from build123d import *

# Parameters (mm, degrees)
SKETCH1_W           = 33
SKETCH1_H           = 28
BOSS_EXTRUDE1_DEPTH = 46
CUT_EXTRUDE1_DEPTH  = 59.318093247
CUT_EXTRUDE2_START  = -3
CUT_EXTRUDE2_DEPTH  = 27
FILLET2_R           = 12.5
FILLET3_R           = 16.5
FILLET4_R           = 6
SKETCH5_W           = 13
SKETCH5_H           = 23
CUT_EXTRUDE3_DEPTH  = 9
SKETCH6_R           = 6.5
CUT_EXTRUDE4_DEPTH  = 56.592265809
SKETCH7_R           = 1
CUT_EXTRUDE6_DEPTH  = 8
SKETCH8_R           = 1.3
SKETCH8_R_2         = 2.5
CUT_EXTRUDE7_DEPTH  = 2.5


with BuildPart() as part:
    # Sketch1 → Boss-Extrude1 (new body)
    with BuildSketch(Plane.XY):
        Rectangle(SKETCH1_W, SKETCH1_H)
    extrude(amount=BOSS_EXTRUDE1_DEPTH)

    # Sketch2 → Cut-Extrude1 (cut, through all)
    with BuildSketch(Plane(origin=(16.5, 0, 0), x_dir=(0, 0, -1), z_dir=(1, 0, 0))):
        with BuildLine():
            Line((-46, 2), (-46, -14))
            Line((-46, -14), (-5, -14))
            add(Edge.make_bspline(
                [(-5, -14), (-24.903930892, -4.26145895), (-46, 2)],
                knots=[0, 0, 0, 1, 1, 1], degree=2))
        make_face()
    extrude(amount=-CUT_EXTRUDE1_DEPTH, mode=Mode.SUBTRACT)

    # Sketch4 → Cut-Extrude2 (cut)
    with BuildSketch(Plane(origin=(16.5, 0, 0), x_dir=(0, 0, -1), z_dir=(1, 0, 0)).offset(CUT_EXTRUDE2_START)):
        with BuildLine():
            Line((-5, -14), (-2.5, -14))
            Line((-2.5, -14), (-2.5, 3.5))
            Line((-2.5, 3.5), (-40.5, 3.5))
            Line((-40.5, 3.5), (-40.5, 0.301980422))
            add(Edge.make_bspline(
                [(-5, -14), (-22.299705813, -5.535647097), (-40.5, 0.301980422)],
                knots=[0, 0, 0, 1, 1, 1], degree=2))
        make_face()
    extrude(amount=-CUT_EXTRUDE2_DEPTH, mode=Mode.SUBTRACT)

    # Fillet2
    fillet2_edges = [part.edges().sort_by_distance(p)[0] for p in [
        (-13.5, 1.900990211, 40.5),
        (13.5, 1.900990211, 40.5),
    ]]
    fillet(fillet2_edges, radius=FILLET2_R)

    # Fillet3
    fillet3_edges = [part.edges().sort_by_distance(p)[0] for p in [
        (-16.5, 8, 46),
        (16.5, 8, 46),
    ]]
    fillet(fillet3_edges, radius=FILLET3_R - 0.0001)  # a hair under: the kernel refuses the full size

    # Fillet4
    fillet4_edges = [part.edges().sort_by_distance(p)[0] for p in [
        (-16.5, -14, 2.5),
        (16.5, -14, 2.5),
    ]]
    fillet(fillet4_edges, radius=FILLET4_R)

    # Sketch5 → Cut-Extrude3 (cut)
    with BuildSketch(Plane.XZ.offset(-3.5)):
        with Locations((0, 20.5)):
            Rectangle(SKETCH5_W, SKETCH5_H)
    extrude(amount=-CUT_EXTRUDE3_DEPTH, mode=Mode.SUBTRACT)

    # Sketch6 → Cut-Extrude4 (cut, through all)
    with BuildSketch(Plane.XZ.offset(-12.5)):
        with Locations(Location((0, 25.5, 0), (0, 0, 270))):
            Circle(SKETCH6_R)
    extrude(amount=-CUT_EXTRUDE4_DEPTH, mode=Mode.SUBTRACT)

    # Sketch7 → Cut-Extrude6 (cut)
    with BuildSketch(Plane.XZ.offset(-3.5)):
        with Locations(Location((0, 34.052667497, 0), (0, 0, 270))):
            Circle(SKETCH7_R)
        with Locations(Location((0, 6.452667497, 0), (0, 0, 270))):
            Circle(SKETCH7_R)
    extrude(amount=-CUT_EXTRUDE6_DEPTH, mode=Mode.SUBTRACT)

    # Sketch8 → Cut-Extrude7 (cut)
    with BuildSketch(Plane(origin=(0, 0, 0), x_dir=(-1, 0, 0), z_dir=(0, 0, -1))):
        with Locations((-9.5, 0)):
            Circle(SKETCH8_R)
        with Locations((-5, 0)):
            Circle(SKETCH8_R_2)
        with Locations((-0.5, 0)):
            Circle(SKETCH8_R)
    extrude(amount=-CUT_EXTRUDE7_DEPTH, mode=Mode.SUBTRACT)


solid = part.part
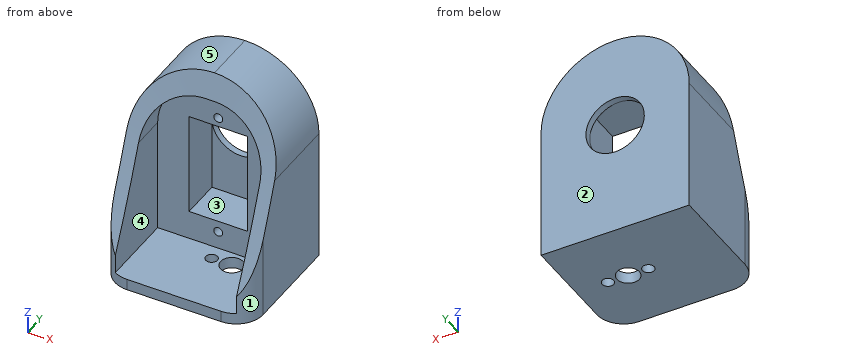
The listing builds one solid part. Answer for the finished solid, in the listing's coordinates (mm). Face numbers are marked on the shaded views. A direction names the side the tool comes from. Give positions to 0.01 mm unless a question says otherwise; leave off trailing zeros. Use a Markdown table: item, result.
1. Section A-A on x = 5 is taken. Count the separate pieces of the cut face and the enclosed holes in it, plus the area to 3 significant figures.
Values follow:
| item | result |
|---|---|
| separate pieces | 3 |
| enclosed holes | 0 |
| area | 300 mm² |
2. For a pull along X with two mould halves and no side action, classify the marked faces 1, 2 and 3 as released by +X, released by -X, zero draft, split by the parting line, or undercut.
Values follow:
| item | result |
|---|---|
| face 1 | released by +X |
| face 2 | zero draft |
| face 3 | undercut |
3. Find the intervals of material crossed by probe 1 along X at (y, z) = (-3.5, 22); probe 2 along X at (y, z) = (13.35, 25.5); probe 3 along Y at (x, z) = (9.5, 1.4), in increasing order. Write a range as from..to.
Values follow:
| item | result |
|---|---|
| probe 1 | x = -16.5..-13.5, 13.5..16.5 |
| probe 2 | x = -16.5..-6.5, 6.5..16.5 |
| probe 3 | y = -14..-1.3, 1.3..14 |
4. Each of these flat-tipped pins is pushed along its axis until it touches: P1, Ø1.6, axis at x = 0, z = 6.45, coming from the -Y side; P2, Ø1, axis at x = -6.5, y = -3, coming from the +Z side; P3, Ø3, axis at x = 9.5, y = 0, coming from the +Z side. Where does it stop, or does it pass through?
Values follow:
| item | result |
|---|---|
| P1 | stops at y = 11.5 |
| P2 | stops at z = 2.5 |
| P3 | stops at z = 43.53 |
5. A tool of negligible diameter and unlimited length cuts with its end or side. For the marked faces 4 and 5, from which of +Z, -Z, +X, -X, +Y, -Y can it reach the whole face along a straight path? Write none if from no direction.
Values follow:
| item | result |
|---|---|
| face 4 | -Y |
| face 5 | +Z, -X, +Y, -Y |
